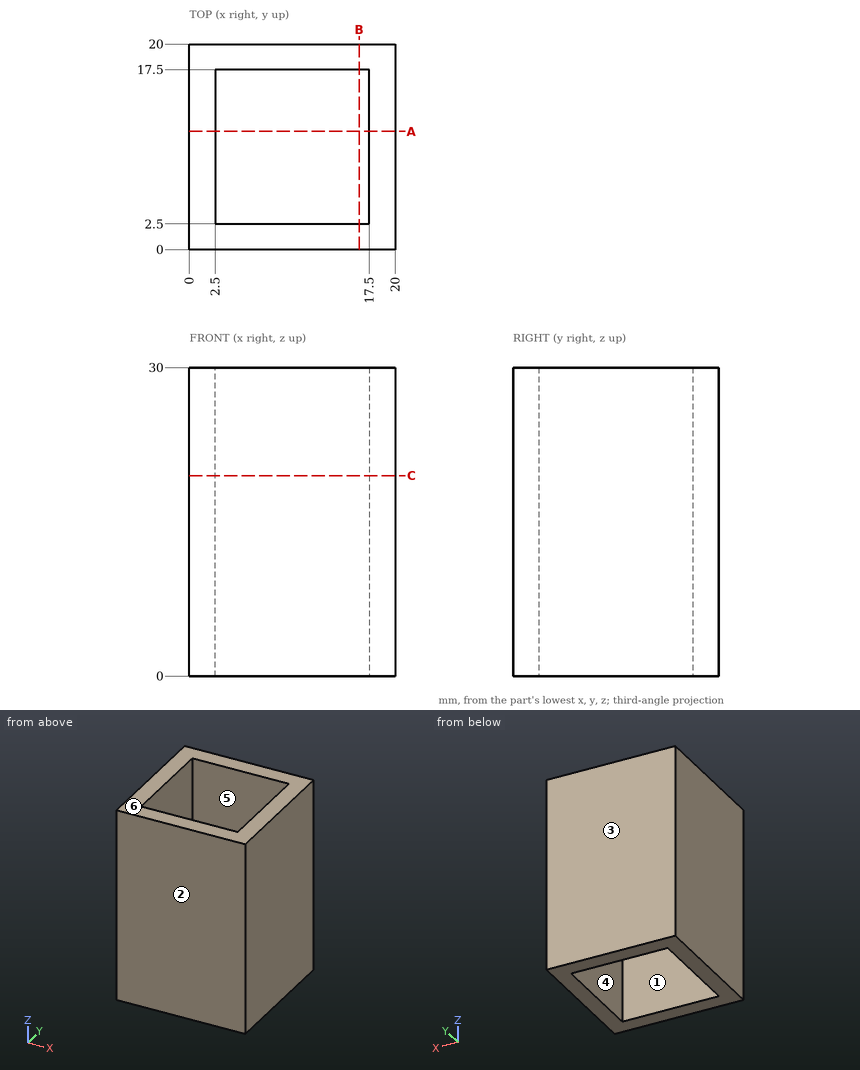
Verification items for this drawing (mm, ordinates from the low corner). A direction names the side the tool comes from. Coordinates: 2 decimals unless noted, no trailing zeros. Loops run counter-clockwise (first coordinate to the right, second up) from the corner with the lowest first, then second, coordinate; pieces in that order, holes last.
Item 1: Go/stop test with a flat-tipped pin: pin 1 Ø6 at (y, z) = (12, 13) entering from -X. Record where the tip stops, or that it passes through.
Item 2: Sectioned sample at A-A, the plane y = 11.5. Record the boundary of the cut face in (x, z).
Item 3: Access from +Z, -Z, +X, -X, +Y, -Y to the whole of each face (thin tool, end or side, straight path). Record for the marked faces 1 and 2.
Item 4: Thickness scan on line 1 (X direction, y = 3.25, z = 24.5). Record the ranges inside material, lowest first.
Item 5: Release check for a two-part mould opening along Y. For the marked faces 3, 4, 5 and 6 record: released by +Y, released by -Y, zero draft, split by the parting line, or undercut.
Item 6: Sectioned sample at C-C, the plane z = 19.5. Record the boundary of the cut face in (x, y), then the cut area to 3 significant figures.
Check result:
1. pin 1: stops at x = 0
2. outline: (0, 0) - (2.5, 0) - (2.5, 30) - (0, 30) - close; (17.5, 0) - (20, 0) - (20, 30) - (17.5, 30) - close
3. face 1: +Z, -Z
3. face 2: +Z, -Z, +X, -X, -Y
4. line 1: x = 0 to 2.5, 17.5 to 20
5. face 3: released by +Y
5. face 4: undercut
5. face 5: undercut
5. face 6: zero draft
6. outline: (0, 0) - (20, 0) - (20, 20) - (0, 20) - close; hole (2.5, 2.5) - (17.5, 2.5) - (17.5, 17.5) - (2.5, 17.5) - close
6. area: 175 mm2
